CAD build for the part. Positions are in the model's coordinates, mm. Face numbers are marked on the shaded views. A direction names the side the tool comes from. Give positions to 0.01 mm unless a question says otherwise; leave off trailing zeros. Write each loop counter-clockwise with the first axis right and the second up, starting at its lowest first coordinate (ties: lowest second). Pieces come first, ordered by that corner, then holes. Notation, with made-up numbers: (-33.75, 59) - (-1.75, 59) arc R24 cw to (-1.75, 92) - close; hole circle Ø3 at (16.5, 5). An arc over 180 degrees is marked (long way). Answer as a JSON object with one key per item and string values.
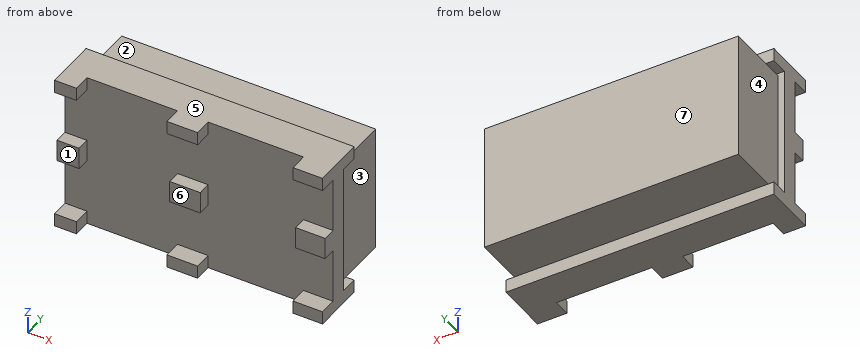
from build123d import *

# Parameters (mm, degrees)
SKETCH1_W               = 104.14
SKETCH1_H               = 3.81
BOSS_EXTRUDE1_DEPTH     = 5.08
BOSS_EXTRUDE1_2_DEPTH   = 5.08
SKETCH2_W               = 104.14
SKETCH2_H               = 45.72
BOSS_EXTRUDE2_DEPTH     = 5.08
SKETCH3_W               = 104.14
SKETCH3_H               = 3.81
BOSS_EXTRUDE3_DEPTH     = 5.08
SKETCH4_W               = 104.14
SKETCH4_H               = 6.3754
BOSS_EXTRUDE4_DEPTH     = 3.81
CUT_EXTRUDE1_DEPTH      = 71.949706835
CUT_EXTRUDE1_DEPTH_BACK = 71.949706835
SKETCH5_W               = 26.368614406
SKETCH5_H               = 5.08
SKETCH5_W_2             = 27.756452018
SKETCH5_W_3             = 30.305435834
SKETCH5_H_2             = 26.045246771
SKETCH6_W               = 73.974469525
SKETCH6_H               = 37.113471059
BOSS_EXTRUDE5_DEPTH     = 19.05


with BuildPart() as part:
    # Sketch1 → Boss-Extrude1 (new body)
    with BuildSketch(Plane(origin=(0, 0, 0), x_dir=(1, 0, 0), z_dir=(0, 1, 0))):
        with Locations((0, -20.955)):
            Rectangle(SKETCH1_W, SKETCH1_H)
    extrude(amount=BOSS_EXTRUDE1_DEPTH)



with BuildPart() as body_2:
    # Sketch1 → Boss-Extrude1 2 (new body)
    with BuildSketch(Plane(origin=(0, 0, 0), x_dir=(1, 0, 0), z_dir=(0, 1, 0))):
        with Locations((0, 20.955)):
            Rectangle(SKETCH1_W, SKETCH1_H)
    extrude(amount=BOSS_EXTRUDE1_2_DEPTH)


with BuildPart() as part_1:
    add(part.part)

    add(body_2.part)  # Boss-Extrude2 merges body 2
    # Sketch2 → Boss-Extrude2 (add)
    with BuildSketch(Plane(origin=(0, 5.08, 0), x_dir=(1, 0, 0), z_dir=(0, 1, 0))):
        Rectangle(SKETCH2_W, SKETCH2_H)
    extrude(amount=BOSS_EXTRUDE2_DEPTH)

    # Sketch3 → Boss-Extrude3 (add)
    with BuildSketch(Plane(origin=(0, 10.16, 0), x_dir=(1, 0, 0), z_dir=(0, 1, 0))):
        with Locations((0, 20.955)):
            Rectangle(SKETCH3_W, SKETCH3_H)
        with Locations((0, -20.955)):
            Rectangle(SKETCH3_W, SKETCH3_H)
    extrude(amount=BOSS_EXTRUDE3_DEPTH)

    # Sketch4 → Boss-Extrude4 (add)
    with BuildSketch(Plane.XZ.offset(-5.08)):
        Rectangle(SKETCH4_W, SKETCH4_H)
    extrude(amount=BOSS_EXTRUDE4_DEPTH)

    # Sketch5 → Cut-Extrude1 (cut, two sides: drawn at the far end of the back side and taken through both)
    with BuildSketch(Plane.XY.offset(22.86).offset(-CUT_EXTRUDE1_DEPTH_BACK)):
        with Locations((-32.471537131, 2.54)):
            Rectangle(SKETCH5_W, SKETCH5_H)
        with Locations((3.530263491, 2.54)):
            Rectangle(SKETCH5_W_2, SKETCH5_H)
        with Locations((41.178408022, 7.587510726)):
            Rectangle(SKETCH5_W_3, SKETCH5_H_2)
    extrude(amount=CUT_EXTRUDE1_DEPTH + CUT_EXTRUDE1_DEPTH_BACK, mode=Mode.SUBTRACT)

    # Sketch6 → Boss-Extrude5 (add)
    with BuildSketch(Plane(origin=(0, 10.16, 0), x_dir=(1, 0, 0), z_dir=(0, 1, 0))):
        with Locations((-13.148391244, 0.168315062)):
            Rectangle(SKETCH6_W, SKETCH6_H)
    extrude(amount=BOSS_EXTRUDE5_DEPTH)


solid = part_1.part
(1) Saw through at D-D, the plane y = 2.25. State how many separate pieces and enclosed holes the cut face has, and give its area (3 significant figures).
Answer key:
{"separate pieces": "9", "enclosed holes": "0", "area": "335 mm²"}
(2) Probe L1, parallel to Z at x = -46.5, y = 2.75; L2, parallel to Z at x = -24, y = 11; L3, parallel to X at y = 21.5, z = 10.5. List the from-to ranges inside material, lowest first. Write a range as [from, to].
Answer key:
{"L1": "z = [-22.86, -19.05], [-3.19, 3.19], [19.05, 22.86]", "L2": "z = [-22.86, -19.05], [-18.73, 18.39], [19.05, 22.86]", "L3": "x = [-50.14, 23.84]"}
(3) Pull direction Z, two halves, no side cores. Call the marked faces 5, 6 and 7: pulls with the +Z half, pulls with the -Z half, needs draft (parallel to the pull), parting line crosses it, or undercut.
Answer key:
{"face 5": "pulls with the +Z half", "face 6": "undercut", "face 7": "needs draft"}
(4) 3-axis set-ups, long thin cutter, end or side, ignore diameter. For the marked faces 1, 2, 3 and 4: which of +Z, -Z, +X, -X, +Y, -Y reach the whole face in a straight line?
Answer key:
{"face 1": "+X, -X, -Y", "face 2": "+X, -X, +Y", "face 3": "+X, +Y", "face 4": "-X, +Y"}
(5) Saw through at B-B, the plane z = 2. Give the cut face in (x, y), and give its area (3 significant figures).
Answer key:
{"outline": "(-52.07, 1.27) - (-45.66, 1.27) - (-45.66, 5.08) - (-19.29, 5.08) - (-19.29, 1.27) - (-10.35, 1.27) - (-10.35, 5.08) - (17.41, 5.08) - (17.41, 1.27) - (26.03, 1.27) - (26.03, 10.16) - (23.84, 10.16) - (23.84, 29.21) - (-50.14, 29.21) - (-50.14, 10.16) - (-52.07, 10.16) - close", "area": "1,900 mm²"}
(6) Saw through at A-A, the plane x = -12. Give the cut face in (y, z), and give its area (3 significant figures).
Answer key:
{"outline": "(0, -22.86) - (15.24, -22.86) - (15.24, -19.05) - (10.16, -19.05) - (10.16, -18.73) - (29.21, -18.73) - (29.21, 18.39) - (10.16, 18.39) - (10.16, 19.05) - (15.24, 19.05) - (15.24, 22.86) - (0, 22.86) - (0, 19.05) - (5.08, 19.05) - (5.08, 3.19) - (1.27, 3.19) - (1.27, -3.19) - (5.08, -3.19) - (5.08, -19.05) - (0, -19.05) - close", "area": "1,040 mm²"}
(7) Flat gauge pins, fed straight in: P1, Ø4, axis at x = -32.5, z = 21.5, coming from the +Y side; P2, Ø10, axis at y = 18.5, z = 1.5, coming from the -X side; P3, Ø1, axis at x = -31, z = -15, coming from the -Y side. Where does each tip first touch, or does it go through?
Answer key:
{"P1": "stops at y = 15.24", "P2": "stops at x = -50.14", "P3": "stops at y = 5.08"}
(8) Saw through at C-C, the plane y = 19.5. Give the cut face in (x, z).
Answer key:
{"outline": "(-50.14, -18.73) - (23.84, -18.73) - (23.84, 18.39) - (-50.14, 18.39) - close"}
